Part model, mm, in its own coordinate system. Face numbers are marked on the shaded views. A direction names the side the tool comes from. Give positions to 0.01 mm unless a question says otherwise; leave off trailing zeros. Order: outer loops, then holes, each group sorted by start corner. A loop starts at its lowest first (then second) coordinate and runs counter-clockwise, first axis right, second up. Notation, with made-up numbers: (7, 9.25) - (54, 9.25) arc R19 ccw to (54, 29.25) - close; hole circle Ø11 at (-11, 72.5). An arc over 180 degrees is marked (long way). One line per item, written item: value.
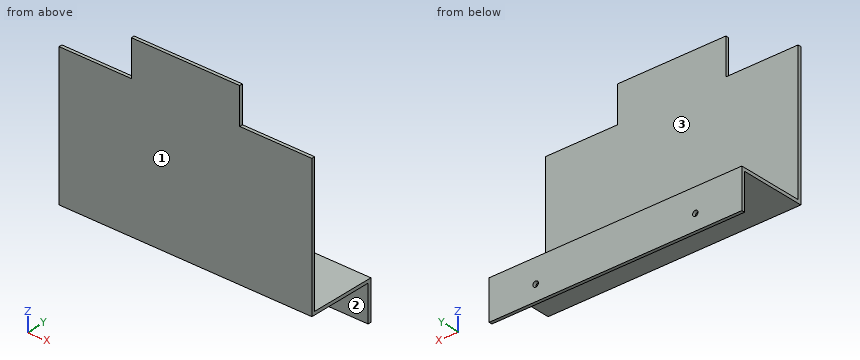
Autodesk Inventor part; units mm, degrees
ref_plane "YZ Plane" through (0, 0, 0) normal (1, 0, 0) x (0, 1, 0)
ref_plane "XZ Plane" through (0, 0, 0) normal (0, 1, 0) x (-1, 0, 0)
ref_plane "XY Plane" through (0, 0, 0) normal (0, 0, 1) x (1, 0, 0)
sketch "Sketch1" plane through (0, 0, 0) normal (1, 0, 0) x (0, 1, 0)
  line L0 (0, 0) -> (2.286, 0)
  line L1 (2.286, 0) -> (2.286, -25.4)
  line L2 (2.286, -25.4) -> (0, -25.4)
  line L3 (0, -25.4) -> (0, 0)
  line L4 (0, 0) -> (-45.974, 0)
  line L5 (-45.974, 0) -> (-45.974, 123.825)
  line L6 (-45.974, 123.825) -> (-43.688, 123.825)
  line L7 (-43.688, 123.825) -> (-43.688, 0)
  line L8 (-45.974, 0) -> (-45.974, 2.286)
  line L9 (-45.974, 2.286) -> (2.286, 2.286)
  line L10 (2.286, 2.286) -> (2.286, 0)
  point P0 (-43.688, 2.286)
  dimension "d0" = 25.4
  dimension "d1" = 2.286
  dimension "d4" = 2.286
  dimension "d5" = 2.286
extrude "Extrusion1" add sketch "Sketch1" along normal blind 177.8
sketch "Sketch2" plane through (0, -43.688, 123.825) normal (0, 1, 0) x (1, 0, 0)
  line L0 (0, 0) -> (177.8, 0)
  line L1 (0, 0) -> (50.8, 0)
  line L2 (50.8, 0) -> (50.8, 25.4)
  line L3 (50.8, 25.4) -> (0, 25.4)
  line L4 (0, 25.4) -> (0, 0)
  line L5 (177.8, 0) -> (127, 0)
  line L6 (127, 0) -> (127, 25.4)
  line L7 (127, 25.4) -> (177.8, 25.4)
  line L8 (177.8, 25.4) -> (177.8, 0)
  point P0 (0, 123.825)
  point P1 (50.8, 0)
  point P2 (127, 0)
  dimension "d8" = 50.8
  dimension "d9" = 25.4
  dimension "d10" = 50.8
extrude "Extrusion2" cut sketch "Sketch2" against normal blind 177.8
sketch "Sketch4" plane through (0, 2.286, 2.286) normal (0, 1, 0) x (1, 0, 0)
  line L0 (0, 2.286) -> (0, 27.686)
  line L1 (0, 16.6049) -> (177.8, 16.7157)
  line L2 (177.8, 27.686) -> (177.8, 0)
  circle A0 centre (32.7282, 16.6253) radius 1.905
  line L3 (0, 27.686) -> (177.8, 27.686)
  line L4 (0, 0) -> (177.8, 0)
  line L5 (177.8, 27.686) -> (145.0594, 27.686)
  line L6 (145.0594, 27.686) -> (145.0594, 0)
  line L7 (145.0594, 0) -> (177.8, 0)
  line L8 (177.8, 0) -> (177.8, 27.686)
  circle A1 centre (145.0594, 16.6953) radius 1.905
  dimension "d13" = 3.81
  dimension "d14" = 32.7406
  dimension "d15" = 3.81
extrude "Extrusion3" cut sketch "Sketch4" against normal blind 177.8 contours A0 L1 | L1 A0 | A1 L1 L6 | L6 L1 A1 | L1 L6 A1 | L1 A1 L6
properties part number "Plate"
1) Wall check: line 1 along Z through (x, y) = (12, -32); line 2 along Y through (x, z) = (67, 104.5). Give the ranges that are in metal, low to high. Write a range as [from, to].
Answer:
line 1: z = [0, 2.29]
line 2: y = [-45.97, -43.69]
2) Which spindle directions (+Z, -Z, +X, -X, +Y, -Y) get a long thin tool onto all of the face, cutting with end or side? Do the marked faces 1, 2 and 3. Say none if no direction does.
Answer:
face 1: +Z, -Z, +X, -X, -Y
face 2: -Z, +X, -X, -Y
face 3: +Z, +X, -X, +Y
3) Slice it at C-C on z = 79. Write the cut outline in (x, y).
Answer:
outline: (0, -45.97) - (177.8, -45.97) - (177.8, -43.69) - (0, -43.69) - close
4) Slice it at A-A on x = 123.5. Write the cut outline in (y, z) (3 decimals), then the cut area to 3 significant figures.
Answer:
outline: (-45.974, 0) - (0, 0) - (0, -25.4) - (2.286, -25.4) - (2.286, 2.286) - (-43.688, 2.286) - (-43.688, 123.825) - (-45.974, 123.825) - close
area: 446 mm2
5) Slice it at B-B on y = -17. Write the cut outline in (x, z).
Answer:
outline: (0, 0) - (177.8, 0) - (177.8, 2.29) - (0, 2.29) - close
6) Drop flat-ended pins along their axis: P1, Ø1, axis at x = 62.5, y = -14, coming from the +Z side; P2, Ø1.8, axis at x = 148, y = -44.5, coming from the +Z side (3 decimals); P3, Ø3, axis at x = 32.73, z = -14.34, coming from the -Y side; P4, Ø2.5, axis at y = -44.5, z = 110, coming from the +X side. Give the stop position or say it passes through.
Answer:
P1: stops at z = 2.29
P2: stops at z = 98.425
P3: passes through
P4: stops at x = 127
